Drawing for the job (mm, zero at the part's lowest x, y, z). A direction names the side the tool comes from. Give positions to 0.01 mm unless a question says otherwise; leave off trailing zeros. Write each loop counter-clockwise with the first axis right and the second up, starting at its lowest first coordinate (ties: lowest second). Pieces come first, ordered by that corner, then holes. Notation, with made-up numbers: (39.5, -36) - (98.5, -36) arc R22 ccw to (98.5, -7) - close; hole circle Ø2 at (66, 51.25). An arc over 180 degrees is marked (long way). Use CSV: the item, a comma, the result in double quotes.
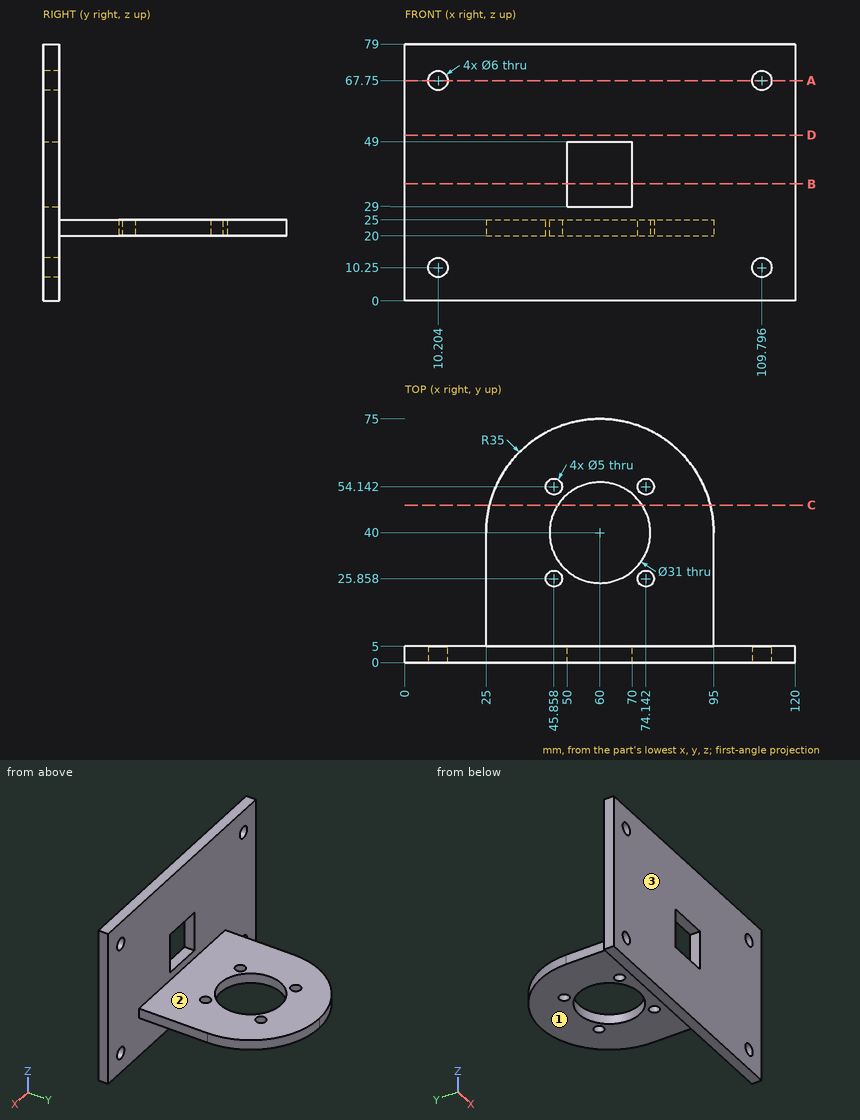
(1) Saw through at A-A, the plane z = 67.75. List the corners of the cut face in (x, y).
Checked values:
outline,"(0, 0) - (7.2, 0) - (7.2, 5) - (0, 5) - close; (13.2, 0) - (106.8, 0) - (106.8, 5) - (13.2, 5) - close; (112.8, 0) - (120, 0) - (120, 5) - (112.8, 5) - close"
(2) Saw through at C-C, the plane y = 48.5. List the corners of the cut face in (x, z).
Checked values:
outline,"(26.05, 20) - (47.04, 20) - (47.04, 25) - (26.05, 25) - close; (72.96, 20) - (93.95, 20) - (93.95, 25) - (72.96, 25) - close"
(3) Flat gauge pins, fed straight in: P1, Ø10, axis at x = 78, y = 28.5, coming from the -Z side; P2, Ø1, axis at x = 94, y = 48, coming from the +Z side; P3, Ø6, axis at x = 57.5, z = 50, coming from the +Y side. Where does each tip first touch, or does it go through?
Checked values:
P1,"stops at z = 20"
P2,"stops at z = 25"
P3,"stops at y = 5"
(4) Wall check: probe 1 along Z at (x, y) = (93.5, 27.5); probe 2 along Y at (x, z) = (41, 15.5); probe 3 along X at (y, z) = (51, 23) (1 decimal). Give the ranges that are in metal, low to high. Write a range as [from, to].
Checked values:
probe 1,"z = [20, 25]"
probe 2,"y = [0, 5]"
probe 3,"x = [26.8, 49.1], [70.9, 93.2]"
(5) 3-axis set-ups, long thin cutter, end or side, ignore diameter. For the marked faces 1, 2 and 3: which of +Z, -Z, +X, -X, +Y, -Y reach the whole face in a straight line?
Checked values:
face 1,"-Z, +X, -X, +Y"
face 2,"+Z, +X, -X, +Y"
face 3,"+Z, -Z, +X, -X, -Y"
(6) Saw through at B-B, the plane z = 36. List the corners of the cut face in (x, y), then the cut area to 3 significant figures.
Checked values:
outline,"(0, 0) - (50, 0) - (50, 5) - (0, 5) - close; (70, 0) - (120, 0) - (120, 5) - (70, 5) - close"
area,"500 mm^2"
(7) Saw through at D-D, the plane z = 51. List the corners of the cut face in (x, y), then the cut area to 3 significant figures.
Checked values:
outline,"(0, 0) - (120, 0) - (120, 5) - (0, 5) - close"
area,"600 mm^2"
